```python
from build123d import *

# Parameters (mm, degrees)
F0_W     = 247.65
F0_H     = 95.25
F1_DEPTH = 6.35
F2_SIZE  = 3.175
F3_W     = 241.3
F3_H     = 88.9
F4_DEPTH = 3.175
F5_W     = 247.65
F5_H     = 95.25
F6_DEPTH = 3.175
F8_DEPTH = 3.175


with BuildPart() as f1:
    # F0 (on Front) → F1 (new body)
    with BuildSketch(Plane.XZ):
        with Locations((92.016742897, 47.625)):
            Rectangle(F0_W, F0_H)
    extrude(amount=F1_DEPTH)

    # F2
    f2_edges = [f1.edges().sort_by_distance(p)[0] for p in [
        (92.016743, -6.35, 95.25),
        (-31.808257, -6.35, 47.625),
        (92.016743, -6.35, 0),
        (215.841743, -6.35, 47.625),
    ]]
    chamfer(f2_edges, length=F2_SIZE)

    # F3 (on face) → F4 (join)
    with BuildSketch(Plane(origin=(0, 0, 0), x_dir=(-1, 0, 0), z_dir=(0, 1, 0))):
        with Locations((-92.016742897, 47.625)):
            Rectangle(F3_W, F3_H)
    extrude(amount=F4_DEPTH)

    # F5 (on face) → F6 (join)
    with BuildSketch(Plane(origin=(0, 3.175, 0), x_dir=(-1, 0, 0), z_dir=(0, 1, 0))):
        with Locations((-92.016742897, 47.625)):
            Rectangle(F5_W, F5_H)
    extrude(amount=F6_DEPTH)

    # F7 (on face) → F8 (cut)
    with BuildSketch(Plane(origin=(0, 6.35, 0), x_dir=(-1, 0, 0), z_dir=(0, 1, 0))):
        Polygon((-203.1155885079, 63.506246084), (-203.115601368, 63.5), (-203.141742897, 50.8031365043), (-203.141742897, 38.1062460972), (-200.2356058372, 38.1002626615), (-200.0943615794, 50.7999993861), (31.808257103, 50.5612678826), (31.808257103, 63.0225621771), align=None)
        Polygon((-203.141742897, 50.8031365043), (-203.115601368, 63.5), (-203.141742897, 63.5), align=None)
    extrude(amount=-F8_DEPTH, mode=Mode.SUBTRACT)


solid = f1.part
```
Source: CAD feature listing. Evaluate the final solid. Frame: model axes, mm. Give positions to 0.01 mm unless a question says otherwise; leave off trailing zeros. Write each loop counter-clockwise with the first axis right and the second up, starting at its lowest first coordinate (ties: lowest second). Pieces come first, ordered by that corner, then holes. Notation, with made-up numbers: (75, -16) - (90, -16) arc R23 cw to (90, 2) - close; hole circle Ø6 at (48.25, 43.25). An arc over 180 degrees is marked (long way). One line per item, written item: value. Start each with the question number.
Q1. Section query A-A, the plane x = -7. Return the cut outline in (y, z) (3 decimals), then the cut area to 3 significant figures.
Q2. Section query B-B, the plane x = 22. Return the cut outline in (y, z) (3 decimals), then the cut area to 3 significant figures.
Q3. First-contact query: pin 1 Ø1 at (y, z) = (-4.5, 45) entering from -X; pin 2 Ø1 at (x, y) = (142.5, 2) entering from +Z (3 decimals); pin 3 Ø1.6 at (y, z) = (1, 59.5) entering from -X. Flat tips, straight axial feed; report the tip coordinate or a pass-through.
Q4. Material intervals for probe 1 along Z at (x, y) = (152, 2.75) (3 decimals); probe 2 along X at (y, z) = (1, 88); probe 3 along Z at (x, y) = (166.5, 5), sorted ascending. Write a range as from..to.
Answer:
1. outline: (-6.35, 3.175) - (-3.175, 0) - (0, 0) - (0, 3.175) - (3.175, 3.175) - (3.175, 0) - (6.35, 0) - (6.35, 50.587) - (3.175, 50.587) - (3.175, 63.074) - (6.35, 63.074) - (6.35, 95.25) - (3.175, 95.25) - (3.175, 92.075) - (0, 92.075) - (0, 95.25) - (-3.175, 95.25) - (-6.35, 92.075) - close
1. area: 1,140 mm2
2. outline: (-6.35, 3.175) - (-3.175, 0) - (0, 0) - (0, 3.175) - (3.175, 3.175) - (3.175, 0) - (6.35, 0) - (6.35, 50.617) - (3.175, 50.617) - (3.175, 63.133) - (6.35, 63.133) - (6.35, 95.25) - (3.175, 95.25) - (3.175, 92.075) - (0, 92.075) - (0, 95.25) - (-3.175, 95.25) - (-6.35, 92.075) - close
2. area: 1,140 mm2
3. pin 1: stops at x = -30.98
3. pin 2: stops at z = 92.075
3. pin 3: stops at x = -28.63
4. probe 1: z = 3.175..92.075
4. probe 2: x = -28.63..212.67
4. probe 3: z = 0..50.77, 63.43..95.25
